Verification items for the finished model (mm, model axes). Coordinates: 2 decimals unless noted, no trailing zeros. Loops run counter-clockwise (first coordinate to the right, second up) from the corner with the lowest first, then second, coordinate; pieces in that order, holes last. Notation, with made-up numbers: (65.25, -28) - (107.25, -28) arc R24 cw to (107.25, -2) - close; hole circle Ø6 at (89, 88.25). An arc over 180 degrees is marked (long way). Answer as CSV lines item,"result". Start each with the question number.
1. Gauge pin test, flat end, axial feed: P1, Ø1.5, axis at x = 6, z = 76.5, coming from the -Y side. Record the tip position at first contact, or that the pin passes through.
2. Cross-section at A-A (x = 6.5). Enter the section's corners in (y, z), plus the area to 3 significant figures.
3. Cross-section at B-B (z = 73.5). Enter the section's corners in (x, y), plus the area to 3 significant figures.
4. Material ranges on line 1 (Z direction, x = 2, y = 2.25); line 2 (Y direction, x = 11.25, z = 49); line 3 (Y direction, x = 5, z = 75), recorded low to high. Write a range as [from, to].
```python
from build123d import *

# Parameters (mm, degrees)
BOSS_EXTRUDE1_DEPTH = 165
SKETCH2_R           = 2
BOSS_EXTRUDE2_DEPTH = 10


with BuildPart() as part:
    # Sketch1 → Boss-Extrude1 (new body)
    with BuildSketch(Plane.XY):
        with BuildLine():
            Line((0, 0), (13, 0))
            Line((13, 0), (13, 5))
            ThreePointArc((13, 5), (6.5, 8), (0, 5))
            Line((0, 5), (0, 0))
        make_face()
    extrude(amount=BOSS_EXTRUDE1_DEPTH)

    # Sketch2 → Boss-Extrude2 (add)
    with BuildSketch(Plane.XY.offset(165)):
        with Locations(Location((6.5, 4, 0), (0, 0, 180))):
            Circle(SKETCH2_R)
    extrude(amount=BOSS_EXTRUDE2_DEPTH)


solid = part.part
```
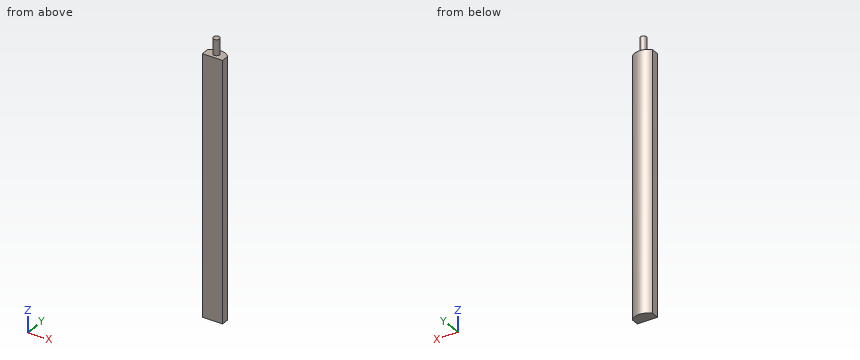
Values follow:
1,P1,"stops at y = 0"
2,outline,"(0, 0) - (8, 0) - (8, 165) - (6, 165) - (6, 175) - (2, 175) - (2, 165) - (0, 165) - close"
2,area,"1,360 mm²"
3,outline,"(0, 0) - (13, 0) - (13, 5) arc R8.54 ccw to (0, 5) - close"
3,area,"92.1 mm²"
4,line 1,"z = [0, 165]"
4,line 2,"y = [0, 6.56]"
4,line 3,"y = [0, 7.87]"
